Geometry: final body of the model. Coordinates: model frame, mm. Give positions to 0.01 mm unless a question says otherwise; leave off trailing zeros. Write each loop counter-clockwise with the first axis right and the second up, starting at its lowest first coordinate (ties: lowest second). Pieces come first, ordered by that corner, then holes. Notation, with made-up numbers: (-31, -26.75) -> (4, -26.75) arc R20 cw to (4, 11.25) -> close; hole circle Ø4 at (57, 47.5). An arc over 180 degrees is marked (long way). Answer in a Markdown table with one row per item. Add a question column.
Item 1: Section query B-B on y = 115.5. Output: boundary loops of the cut face in (x, z).
Item 2: Section query C-C on x = 3.5. Output: boundary loops of the cut face in (y, z), plus the area to 3 significant figures.
Item 3: Section query A-A on z = 6.5. Output: boundary loops of the cut face in (x, y).
Item 4: Section query D-D on x = -91.5. Output: boundary loops of the cut face in (y, z).
Item 5: First-contact query: P1, Ø1.8, axis at x = -170, y = 66, coming from the +Z side; P2, Ø4, axis at x = -135, z = 4, coming from the +Y side; P3, Ø3, axis at x = -189, z = 1, coming from the +Y side. Flat tips, straight axial feed; report the tip coordinate or a pass-through.
Item 6: Material intervals for probe 1 along Y at (x, z) = (-171, 1); probe 2 along Y at (x, z) = (-204, 5.25); probe 3 along X at (y, z) = (90, 4.5), sorted ascending. Write a range as from..to.
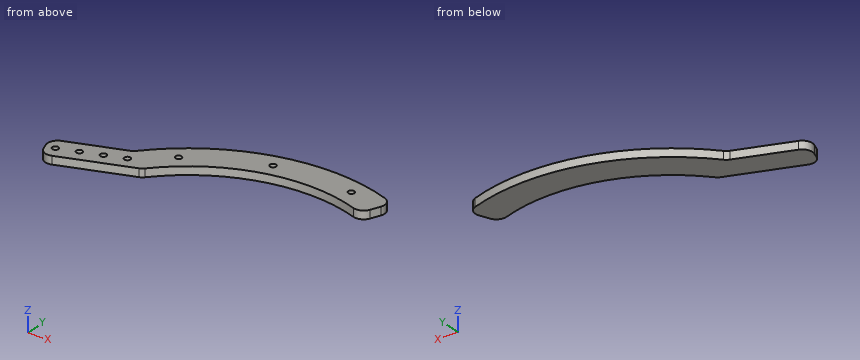
```python
from build123d import *

# Parameters (mm, degrees)
BOSS_EXTRUDE1_DEPTH = 8
SKETCH2_R           = 3
CUT_EXTRUDE1_DEPTH  = 7.8
FILLET1_R           = 10


with BuildPart() as part:
    # Sketch1 → Boss-Extrude1 (new body)
    with BuildSketch(Plane.XY):
        with BuildLine():
            Line((-132.022045573, 65.789710007), (-212.176223927, 37.5))
            Line((-212.176223927, 37.5), (-220.823144233, 61.999607532))
            Line((-220.823144233, 61.999607532), (-154.813820882, 85.297015774))
            ThreePointArc((-154.813820882, 85.297015774), (-54.334940348, 146.616935984), (62.982038035, 136.980306335))
            Line((62.982038035, 136.980306335), (51.384993515, 109.312481006))
            ThreePointArc((51.384993515, 109.312481006), (-47.408251439, 117.427537553), (-132.022045573, 65.789710007))
        make_face()
    extrude(amount=BOSS_EXTRUDE1_DEPTH)

    # Sketch2 → Cut-Extrude1 (cut)
    with BuildSketch(Plane.XY.offset(8)):
        with Locations((-208.012771078, 52.745184826)):
            Circle(SKETCH2_R)
        with Locations((-189.152964406, 59.40158718)):
            Circle(SKETCH2_R)
        with Locations((-170.293157734, 66.057989535)):
            Circle(SKETCH2_R)
        with Locations((-151.433351063, 72.71439189)):
            Circle(SKETCH2_R)
        with Locations((25.722042378, 132.968245202)):
            Circle(SKETCH2_R)
        with Locations((-50.828871081, 131.842192364)):
            Circle(SKETCH2_R)
        with Locations((-119.723860621, 98.45370988)):
            Circle(SKETCH2_R)
    extrude(amount=-CUT_EXTRUDE1_DEPTH, mode=Mode.SUBTRACT)

    # Fillet1
    fillet1_edges = [part.edges().sort_by_distance(p)[0] for p in [
        (-220.823144233, 61.999607532, 4),
        (-154.813820882, 85.297015774, 4),
        (62.982038035, 136.980306335, 4),
        (51.384993515, 109.312481006, 4),
        (-132.022045573, 65.789710007, 4),
        (-212.176223927, 37.5, 4),
    ]]
    fillet(fillet1_edges, radius=FILLET1_R)


solid = part.part
```
Findings below:
| question | item | result |
|---|---|---|
| 1 | outline | (-122.1, 0) -> (-54.75, 0) -> (-54.75, 8) -> (-122.1, 8) -> close; (33.82, 0) -> (53.4, 0) -> (53.4, 8) -> (33.82, 8) -> close |
| 2 | outline | (121.14, 0) -> (151.24, 0) -> (151.24, 8) -> (121.14, 8) -> close |
| 2 | area | 241 mm^2 |
| 3 | outline | (-217.49, 52.57) -> (-215.5, 46.93) arc R10 ccw to (-202.75, 40.83) -> (-134.51, 64.91) arc R10 ccw to (-130.34, 67.72) arc R160 cw to (42.6, 112.7) arc R10 ccw to (55.14, 118.26) -> (59.01, 127.5) arc R10 ccw to (53.13, 140.79) arc R190 ccw to (-153.13, 87.24) arc R10 cw to (-157.31, 84.42) -> (-211.39, 65.33) arc R10 ccw to start; hole circle Ø6 at (-208.01, 52.75); hole circle Ø6 at (-189.15, 59.4); hole circle Ø6 at (-170.29, 66.06); hole circle Ø6 at (-151.43, 72.71); hole circle Ø6 at (-119.72, 98.45); hole circle Ø6 at (-50.83, 131.84); hole circle Ø6 at (25.72, 132.97) |
| 4 | outline | (99.71, 0) -> (133.6, 0) -> (133.6, 8) -> (99.71, 8) -> close |
| 5 | P1 | stops at z = 0.2 |
| 5 | P2 | stops at y = 106.96 |
| 5 | P3 | stops at y = 73.76 |
| 6 | probe 1 | y = 52.03..63.14, 68.97..79.58 |
| 6 | probe 2 | y = 40.48..67.94 |
| 6 | probe 3 | x = -150.65..-106.13 |
